Source: CAD feature listing. Evaluate the final solid. Frame: model axes, mm. A direction names the side the tool comes from. Give positions to 0.01 mm unless a question says otherwise; leave off trailing zeros. Order: outer loops, then holes, each group sorted by start corner. A loop starts at its lowest first (then second) coordinate and runs counter-clockwise, first axis right, second up. Notation, with made-up numbers: M 20,51 L 46,51 A17 cw 46,82 Z; hole C 79.5,-19 d6. An arc over 180 degrees is marked long. Return JSON: item names as keys, results as strings.
from build123d import *

# Parameters (mm, degrees)
SKETCH1_W             = 20
SKETCH1_H             = 25
BOSS_EXTRUDE1_DEPTH   = 20
BOSS_EXTRUDE1_2_DEPTH = 20
SKETCH1_3_W           = 20
SKETCH1_3_H           = 25
BOSS_EXTRUDE2_DEPTH   = 28
SKETCH2_W             = 60
SKETCH2_H             = 9
CUT_EXTRUDE1_DEPTH    = 20
CUT_EXTRUDE2_DEPTH    = 71.774289117
SKETCH4_W             = 15
SKETCH4_H             = 20
SKETCH4_W_2           = 5
CUT_EXTRUDE3_DEPTH    = 17.5
CUT_EXTRUDE5_DEPTH    = 22.5
SKETCH7_R             = 2.55
CUT_EXTRUDE6_DEPTH    = 71.774289117


with BuildPart() as part:
    # Sketch1 → Boss-Extrude1 (new body)
    with BuildSketch(Plane(origin=(0, 0, 0), x_dir=(1, 0, 0), z_dir=(0, 1, 0))):
        with Locations((10, 12.5)):
            Rectangle(SKETCH1_W, SKETCH1_H)
    extrude(amount=BOSS_EXTRUDE1_DEPTH)



with BuildPart() as body_2:
    # Sketch1 → Boss-Extrude1 2 (new body)
    with BuildSketch(Plane(origin=(0, 0, 0), x_dir=(1, 0, 0), z_dir=(0, 1, 0))):
        with Locations((50, 12.5)):
            Rectangle(SKETCH1_W, SKETCH1_H)
    extrude(amount=BOSS_EXTRUDE1_2_DEPTH)


with BuildPart() as part_1:
    add(part.part)

    add(body_2.part)  # Boss-Extrude2 merges body 2
    # Sketch1<3> → Boss-Extrude2 (add)
    with BuildSketch(Plane(origin=(0, 0, 0), x_dir=(1, 0, 0), z_dir=(0, 1, 0))):
        with Locations((30, 12.5)):
            Rectangle(SKETCH1_3_W, SKETCH1_3_H)
        with Locations((10, 12.5)):
            Rectangle(SKETCH1_3_W, SKETCH1_3_H)
        with Locations((50, 12.5)):
            Rectangle(SKETCH1_3_W, SKETCH1_3_H)
    extrude(amount=-BOSS_EXTRUDE2_DEPTH)

    # Sketch2 → Cut-Extrude1 (cut)
    with BuildSketch(Plane.XY):
        with Locations((30, -20.5)):
            Rectangle(SKETCH2_W, SKETCH2_H)
    extrude(amount=-CUT_EXTRUDE1_DEPTH, mode=Mode.SUBTRACT)

    # Sketch3 → Cut-Extrude2 (cut, through all)
    with BuildSketch(Plane.XY):
        Polygon((0, 20), (0, 0), (17.5, 20), align=None)
        Polygon((42.5, 20), (60, 0), (60, 20), align=None)
    extrude(amount=-CUT_EXTRUDE2_DEPTH, mode=Mode.SUBTRACT)

    # Sketch4 → Cut-Extrude3 (cut)
    with BuildSketch(Plane(origin=(60, 0, 0), x_dir=(0, 0, -1), z_dir=(1, 0, 0))):
        with Locations((12.5, 10)):
            Rectangle(SKETCH4_W, SKETCH4_H)
        with Locations((2.5, 10)):
            Rectangle(SKETCH4_W_2, SKETCH4_H)
    cut_extrude3 = extrude(amount=-CUT_EXTRUDE3_DEPTH, mode=Mode.SUBTRACT)

    # Sketch5 → Cut-Extrude5 (cut)
    with BuildSketch(Plane(origin=(42.5, 0, 0), x_dir=(0, 0, -1), z_dir=(1, 0, 0))):
        with BuildLine():
            ThreePointArc((12.55, 10), (11.803122292, 11.803122292), (10, 12.55))
            Line((10, 12.55), (10, 7.45))
            ThreePointArc((10, 7.45), (11.803122292, 8.196877708), (12.55, 10))
        make_face()
        with BuildLine():
            Line((10, 7.45), (10, 12.55))
            ThreePointArc((10, 12.55), (7.45, 10), (10, 7.45))
        make_face()
    cut_extrude5 = extrude(amount=-CUT_EXTRUDE5_DEPTH, mode=Mode.SUBTRACT)

    # Sketch7 → Cut-Extrude6 (cut, symmetric)
    with BuildSketch(Plane(origin=(0, 0, 0), x_dir=(1, 0, 0), z_dir=(0, 1, 0))):
        with Locations(Location((50, 10.75, 0), (0, 0, 270))):
            Circle(SKETCH7_R)
    cut_extrude6 = extrude(amount=CUT_EXTRUDE6_DEPTH, both=True, mode=Mode.SUBTRACT)

    # Mirror3: Cut-Extrude3, Cut-Extrude5, Cut-Extrude6 across plane
    add(cut_extrude3.mirror(Plane.ZY.offset(-30)), mode=Mode.SUBTRACT)
    add(cut_extrude5.mirror(Plane.ZY.offset(-30)), mode=Mode.SUBTRACT)
    add(cut_extrude6.mirror(Plane.ZY.offset(-30)), mode=Mode.SUBTRACT)


solid = part_1.part
1. Section query C-C (x = 31). Return loops of the section in (y, z).
Evaluation:
{"outline": "M -28,-25 L 0,-25 L 0,0 L -16,0 L -16,-20 L -25,-20 L -25,0 L -28,0 Z"}
2. Ray query, probe 1 along X at (y, z) = (-8, -10.75); probe 2 along Y at (x, z) = (20.5, -16.25); probe 3 along X at (y, z) = (18.5, -7). Return the intervals inside material, ascending.
Evaluation:
{"probe 1": "x = 0 to 7.45, 12.55 to 47.45, 52.55 to 60", "probe 2": "y = -28 to -25, -16 to 0", "probe 3": "x = 17.5 to 20, 40 to 42.5"}
3. Draft query along X for faces 6 (the face through (17.5, 12, -12)), 7 (the face through (30, -9, -25)), 8 (the face through (12.49, -26.48, -11.3)). Return one class per face: pulls with the +X half, pulls with the -X half, needs draft (parallel to the pull), parting line crosses it, or undercut.
Evaluation:
{"face 6": "pulls with the -X half", "face 7": "needs draft", "face 8": "undercut"}
4. Section query B-B (y = -3.5). Return loops of the section in (x, z).
Evaluation:
{"outline": "M 0,-25 L 60,-25 L 60,0 L 0,0 Z; hole C 10,-10.75 d5.1; hole C 50,-10.75 d5.1"}
5. Section query A-A (z = -18). Return loops of the section in (x, y).
Evaluation:
{"outline": "M 0,-28 L 60,-28 L 60,-25 L 0,-25 Z; M 0,-16 L 60,-16 L 60,0 L 42.5,0 L 42.5,20 L 40,20 L 40,0 L 20,0 L 20,20 L 17.5,20 L 17.5,0 L 0,0 Z"}
6. First-contact query: pin 1 (6.5 mm diameter, centred on x = 50, z = -10.75, fed in from +Y); pin 2 (9 mm diameter, centred on x = 8.5, y = 9, fed in from +Z); pin 3 (4.5 mm diameter, centred on x = 10, z = -10.75, fed in from +Y). Flat tips, straight axial feed; report the tip coordinate or a pass-through.
Evaluation:
{"pin 1": "stops at y = 0", "pin 2": "stops at z = -20", "pin 3": "passes through"}
7. Set-up query: faces 1 (the face through (47, 5, -20)), 2 (the face through (13, 5, -20)), 3 (the face through (30, 0, -13)), 4 (the face through (60, -11, -12)), 5 (the face through (30, -20, -20)). Return all of +Z, -Z, +X, -X, +Y, -Y with unobstructed straight access to the full face (end or side cutting, diameter ignored); none if empty.
Evaluation:
{"face 1": "+Z, +X, +Y", "face 2": "+Z, -X, +Y", "face 3": "+Z, -Z, +Y", "face 4": "+Z, -Z, +X, +Y, -Y", "face 5": "+Z, +X, -X"}
8. Section query D-D (z = -21.25). Return loops of the section in (x, y), then the cut area to 3 significant figures.
Evaluation:
{"outline": "M 0,-28 L 60,-28 L 60,0 L 42.5,20 L 40,20 L 40,0 L 20,0 L 20,20 L 17.5,20 L 0,0 Z", "area": "2,130 mm^2"}
